from build123d import *

# Parameters (mm, degrees)
CROQUIS1_R              = 1
CROQUIS1_W              = 3
CROQUIS1_H              = 5.5
CROQUIS1_W_2            = 5.5
CROQUIS1_H_2            = 3
SALIENTE_EXTRUIR1_DEPTH = 3


with BuildPart() as part:
    # Croquis1 → Saliente-Extruir1 (new body)
    with BuildSketch(Plane(origin=(0, 0, 0), x_dir=(1, 0, 0), z_dir=(0, 1, 0))):
        with BuildLine():
            Line((-39, -32.5), (39, -32.5))
            ThreePointArc((39, -32.5), (39.707106781, -32.207106781), (40, -31.5))
            Line((40, -31.5), (40, 31.5))
            ThreePointArc((40, 31.5), (39.707106781, 32.207106781), (39, 32.5))
            Line((39, 32.5), (-39, 32.5))
            ThreePointArc((-39, 32.5), (-39.707106781, 32.207106781), (-40, 31.5))
            Line((-40, 31.5), (-40, -31.5))
            ThreePointArc((-40, -31.5), (-39.707106781, -32.207106781), (-39, -32.5))
        make_face()
        with Locations(Location((-36.5, 29, 0), (0, 0, 270))):
            Circle(CROQUIS1_R, mode=Mode.SUBTRACT)
        with Locations(Location((-36.5, -29, 0), (0, 0, 270))):
            Circle(CROQUIS1_R, mode=Mode.SUBTRACT)
        with Locations(Location((36.5, -29, 0), (0, 0, 90))):
            Circle(CROQUIS1_R, mode=Mode.SUBTRACT)
        with Locations(Location((36.5, 29, 0), (0, 0, 90))):
            Circle(CROQUIS1_R, mode=Mode.SUBTRACT)
        with Locations(Location((-22, 25.3, 0), (0, 0, 270))):
            Circle(CROQUIS1_R, mode=Mode.SUBTRACT)
        with Locations(Location((-22, -24.7, 0), (0, 0, 270))):
            Circle(CROQUIS1_R, mode=Mode.SUBTRACT)
        with Locations(Location((33, 10.5, 0), (0, 0, 270))):
            Circle(CROQUIS1_R, mode=Mode.SUBTRACT)
        with Locations(Location((33, -19.5, 0), (0, 0, 270))):
            Circle(CROQUIS1_R, mode=Mode.SUBTRACT)
        with Locations((-36.5, 20.25)):
            Rectangle(CROQUIS1_W, CROQUIS1_H, mode=Mode.SUBTRACT)
        with Locations((-36.5, -20.25)):
            Rectangle(CROQUIS1_W, CROQUIS1_H, mode=Mode.SUBTRACT)
        with Locations((-27.25, 29)):
            Rectangle(CROQUIS1_W_2, CROQUIS1_H_2, mode=Mode.SUBTRACT)
        with Locations((-27.25, -29)):
            Rectangle(CROQUIS1_W_2, CROQUIS1_H_2, mode=Mode.SUBTRACT)
        with Locations((27.25, -29)):
            Rectangle(CROQUIS1_W_2, CROQUIS1_H_2, mode=Mode.SUBTRACT)
        with Locations((36.5, -20.25)):
            Rectangle(CROQUIS1_W, CROQUIS1_H, mode=Mode.SUBTRACT)
        with Locations((36.5, 20.25)):
            Rectangle(CROQUIS1_W, CROQUIS1_H, mode=Mode.SUBTRACT)
        with Locations((27.25, 29)):
            Rectangle(CROQUIS1_W_2, CROQUIS1_H_2, mode=Mode.SUBTRACT)
    extrude(amount=SALIENTE_EXTRUIR1_DEPTH)


solid = part.part
Design review of the part built by this model. Coordinates are the model's own, in mm. Give positions to 0.01 mm unless a question says otherwise; leave off trailing zeros. Write each loop counter-clockwise with the first axis right and the second up, starting at its lowest first coordinate (ties: lowest second). Pieces come first, ordered by that corner, then holes. Notation, with made-up numbers: M 78.5,54 L 90.5,54 A21 ccw 90.5,76 Z; hole C 1.25,79.25 d10. An arc over 180 degrees is marked long. Answer as a JSON object with one key per item and string values. Group by question number.
1) We need section C-C (x = -36.5). Give the boundary of the cut face in (y, z).
2) We need section A-A (z = 19.5). Give the boundary of the cut face in (x, y), and give its area (3 significant figures).
3) We need section D-D (x = -22). Give the boundary of the cut face in (y, z), and give its area (3 significant figures).
4) We need section B-B (z = 29). Give the boundary of the cut face in (x, y), and give its area (3 significant figures).
5) Clearance check with a flat-ended pin moving along its axis: pin 1 Ø1.2 at (x, z) = (36.5, -29) entering from +Y. State where the tip first meets the part, or that it passes through.
6) For line 1 along Z through (x, y) = (27, 1.2); line 2 along X through (y, z) = (1.55, 19.5); line 3 along X through (y, z) = (1.05, -21), list the stretches that pass through material, from the lowest coordinate up.
7) Mouldability with a two-part tool opening along X and no side actions: class faces 1 (the face through (-30, 1, -29)), 2 (the face through (40, 1, 0)), 3 (the face through (1, 1, -32.5)) as released by +X, released by -X, zero draft, split by the parting line, or undercut.
Answer key:
{
 "1": {"outline": "M 0,-32.5 L 3,-32.5 L 3,-30 L 0,-30 Z; M 0,-28 L 3,-28 L 3,-23 L 0,-23 Z; M 0,-17.5 L 3,-17.5 L 3,17.5 L 0,17.5 Z; M 0,23 L 3,23 L 3,28 L 0,28 Z; M 0,30 L 3,30 L 3,32.5 L 0,32.5 Z"},
 "2": {"outline": "M -40,0 L -38,0 L -38,3 L -40,3 Z; M -35,0 L 32,0 L 32,3 L -35,3 Z; M 34,0 L 35,0 L 35,3 L 34,3 Z; M 38,0 L 40,0 L 40,3 L 38,3 Z", "area": "216 mm²"},
 "3": {"outline": "M 0,-32.5 L 3,-32.5 L 3,-26.3 L 0,-26.3 Z; M 0,-24.3 L 3,-24.3 L 3,23.7 L 0,23.7 Z; M 0,25.7 L 3,25.7 L 3,32.5 L 0,32.5 Z", "area": "183 mm²"},
 "4": {"outline": "M -40,0 L -37.5,0 L -37.5,3 L -40,3 Z; M -35.5,0 L -30,0 L -30,3 L -35.5,3 Z; M -24.5,0 L 24.5,0 L 24.5,3 L -24.5,3 Z; M 30,0 L 35.5,0 L 35.5,3 L 30,3 Z; M 37.5,0 L 40,0 L 40,3 L 37.5,3 Z", "area": "195 mm²"},
 "5": {"pin 1": "passes through"},
 "6": {"line 1": "z = -32.5 to -30.5, -27.5 to 27.5, 30.5 to 32.5", "line 2": "x = -40 to -38, -35 to 32, 34 to 35, 38 to 40", "line 3": "x = -40 to -38, -35 to 35, 38 to 40"},
 "7": {"face 1": "undercut", "face 2": "released by +X", "face 3": "zero draft"}
}
